Part model, mm, in its own coordinate system. Face numbers are marked on the shaded views. Coordinates: 2 decimals unless noted, no trailing zeros. Order: outer loops, then holes, each group sorted by start corner. A loop starts at its lowest first (then second) coordinate and runs counter-clockwise, first axis right, second up.
1) Cut at D-D (x = 49). List the corners of the cut face in (y, z), and give its area (3 significant figures).
2) Pin check, flat tips, straight feed: pin 1 Ø1.3 at (x, y) = (71, 0) entering from +Z; pin 2 Ø8 at (y, z) = (-3, 16) entering from +X; pin 3 Ø9 at (x, z) = (10, 11) entering from -Y; pin 4 Ø2.5 at (x, z) = (53, 11) entering from -Y. Stop position of each tip, or through.
3) Cut at C-C (z = 11). Give the number of separate pieces and of enclosed holes in the cut face, and give its area (3 significant figures).
4) Wall check: L1, parallel to X at y = -13.5, z = 11; L2, parallel to Z at x = 62, y = 0; L3, parallel to X at y = -11, z = 12. Give the ranges that are in metal, low to high.
5) Cut at B-B (y = 22). List the corners of the cut face in (x, z).
6) Cut at A-A (x = 86). List the corners of the cut face in (y, z).
7) Mould opens along Z. For the marked faces 1, 2 and 3 say: +Z half, -Z half, draft (parallel to the pull), parting line (faces both ways), or undercut.
```python
from build123d import *

# Parameters (mm, degrees)
BOSS_EXTRUDE1_DEPTH     = 90
SKETCH2_R               = 7.6
SKETCH2_R_2             = 5.5
CUT_EXTRUDE1_DEPTH      = 90
SKETCH3_R               = 4.1
CUT_EXTRUDE2_DEPTH      = 90
SKETCH10_W              = 1
SKETCH10_H              = 31.35052841
CUT_EXTRUDE_THIN1_DEPTH = 70
SKETCH11_R              = 11.5
CUT_EXTRUDE6_DEPTH      = 7
SKETCH12_R              = 1.95
CUT_EXTRUDE7_DEPTH      = 15
BOSS_EXTRUDE2_START     = -3
SKETCH16_R              = 4.1
BOSS_EXTRUDE2_DEPTH     = 3
FILLET1_R               = 2
SKETCH17_R              = 2.5
CUT_EXTRUDE8_DEPTH      = 30
SKETCH18_W              = 5
SKETCH18_H              = 7.5
CUT_EXTRUDE9_DEPTH      = 44
BOSS_EXTRUDE3_START     = 3
SKETCH19_R              = 3.5
SKETCH19_R_2            = 2.5
BOSS_EXTRUDE3_DEPTH     = 3
CHAMFER1_SIZE           = 3


with BuildPart() as part:
    # Sketch1 → Boss-Extrude1 (new body)
    with BuildSketch(Plane(origin=(0, 0, 0), x_dir=(0, 0, -1), z_dir=(1, 0, 0))):
        with BuildLine():
            Line((-20, -30), (20, -30))
            ThreePointArc((20, -30), (23.535533906, -28.535533906), (25, -25))
            Line((25, -25), (25, 25))
            ThreePointArc((25, 25), (23.535533906, 28.535533906), (20, 30))
            Line((20, 30), (-20, 30))
            ThreePointArc((-20, 30), (-23.535533906, 28.535533906), (-25, 25))
            Line((-25, 25), (-25, -25))
            ThreePointArc((-25, -25), (-23.535533906, -28.535533906), (-20, -30))
        make_face()
    extrude(amount=BOSS_EXTRUDE1_DEPTH)

    # Sketch2 → Cut-Extrude1 (cut)
    with BuildSketch(Plane(origin=(0, 30, 0), x_dir=(1, 0, 0), z_dir=(0, 1, 0))):
        with Locations(Location((10, -11, 0), (0, 0, 270))):
            Circle(SKETCH2_R)
        with Locations(Location((80, -11, 0), (0, 0, 270))):
            Circle(SKETCH2_R)
        with Locations(Location((45, -11, 0), (0, 0, 270))):
            Circle(SKETCH2_R_2)
    extrude(amount=-CUT_EXTRUDE1_DEPTH, mode=Mode.SUBTRACT)

    # Sketch3 → Cut-Extrude2 (cut)
    with BuildSketch(Plane.XY.offset(25)):
        with Locations((20, 0)):
            Circle(SKETCH3_R)
        with Locations((70, 0)):
            Circle(SKETCH3_R)
    extrude(amount=-CUT_EXTRUDE2_DEPTH, mode=Mode.SUBTRACT)

    # Sketch10 → Cut-Extrude-Thin1 (cut)
    with BuildSketch(Plane(origin=(0, 30, 0), x_dir=(1, 0, 0), z_dir=(0, 1, 0))):
        with Locations((10, -26.675264205)):
            Rectangle(SKETCH10_W, SKETCH10_H)
        with Locations((80, -26.675264205)):
            Rectangle(SKETCH10_W, SKETCH10_H)
    extrude(amount=-CUT_EXTRUDE_THIN1_DEPTH, mode=Mode.SUBTRACT)

    # Sketch11 → Cut-Extrude6 (cut)
    with BuildSketch(Plane(origin=(0, -30, 0), x_dir=(-1, 0, 0), z_dir=(0, -1, 0))):
        with Locations(Location((-45, -11, 0), (0, 0, 90))):
            Circle(SKETCH11_R)
    extrude(amount=-CUT_EXTRUDE6_DEPTH, mode=Mode.SUBTRACT)

    # Sketch12 → Cut-Extrude7 (cut)
    with BuildSketch(Plane(origin=(0, -23, 0), x_dir=(-1, 0, 0), z_dir=(0, -1, 0))):
        with Locations(Location((-45, -19, 0), (0, 0, 90))):
            Circle(SKETCH12_R)
        with Locations(Location((-53, -11, 0), (0, 0, 90))):
            Circle(SKETCH12_R)
        with Locations(Location((-45, -3, 0), (0, 0, 90))):
            Circle(SKETCH12_R)
        with Locations(Location((-37, -11, 0), (0, 0, 90))):
            Circle(SKETCH12_R)
    extrude(amount=-CUT_EXTRUDE7_DEPTH, mode=Mode.SUBTRACT)

    # Sketch16 → Boss-Extrude2 (add)
    with BuildSketch(Plane(origin=(0, 0, -25), x_dir=(-1, 0, 0), z_dir=(0, 0, -1)).offset(BOSS_EXTRUDE2_START)):
        with Locations(Location((-70, 0, 0), (0, 0, 180))):
            Circle(SKETCH16_R)
        with Locations(Location((-20, 0, 0), (0, 0, 180))):
            Circle(SKETCH16_R)
    extrude(amount=BOSS_EXTRUDE2_DEPTH)

    # Fillet1
    fillet1_edges = [part.edges().sort_by_distance(p)[0] for p in [
        (65.9, 0, -22),
        (15.9, 0, -22),
    ]]
    fillet(fillet1_edges, radius=FILLET1_R)

    # Sketch17 → Cut-Extrude8 (cut)
    with BuildSketch(Plane(origin=(90, 0, 0), x_dir=(0, 0, -1), z_dir=(1, 0, 0))):
        Circle(SKETCH17_R)
    extrude(amount=-CUT_EXTRUDE8_DEPTH, mode=Mode.SUBTRACT)

    # Sketch18 → Cut-Extrude9 (cut)
    with BuildSketch(Plane(origin=(0, 30, 0), x_dir=(1, 0, 0), z_dir=(0, 1, 0))):
        with Locations((58.5, 0)):
            Rectangle(SKETCH18_W, SKETCH18_H)
    extrude(amount=-CUT_EXTRUDE9_DEPTH, mode=Mode.SUBTRACT)

    # Sketch19 → Boss-Extrude3 (add)
    with BuildSketch(Plane(origin=(90, 0, 0), x_dir=(0, 0, -1), z_dir=(1, 0, 0)).offset(BOSS_EXTRUDE3_START)):
        with Locations(Location((0, 0, 0), (0, 0, 180))):
            Circle(SKETCH19_R)
        Circle(SKETCH19_R_2, mode=Mode.SUBTRACT)
    extrude(amount=-BOSS_EXTRUDE3_DEPTH)

    # Chamfer1
    chamfer1_edges = [part.edges().sort_by_distance(p)[0] for p in [
        (90, 0, -3.5),
    ]]
    chamfer(chamfer1_edges, length=CHAMFER1_SIZE - 0.0001)  # a hair under: the kernel refuses the full size


solid = part.part
```
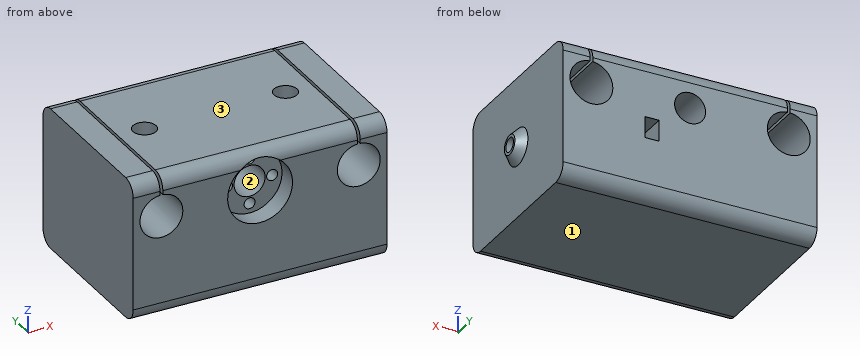
Geometry check:
1. outline: (-30, -20) arc R5 ccw to (-25, -25) - (25, -25) arc R5 ccw to (30, -20) - (30, 7.23) - (-23, 7.23) - (-23, 0.22) - (-30, 0.22) - close; (-29.67, 21.78) - (-23, 21.78) - (-23, 14.77) - (30, 14.77) - (30, 20) arc R5 ccw to (25, 25) - (-25, 25) arc R5 ccw to start
1. area: 2,430 mm2
2. pin 1: stops at z = -22
2. pin 2: stops at x = 90
2. pin 3: passes through
2. pin 4: stops at y = -8
3. separate pieces: 4
3. enclosed holes: 0
3. area: 2,630 mm2
4. L1: x = 0 to 2.4, 17.6 to 35.05, 38.95 to 39.5, 50.5 to 51.05, 54.95 to 72.4, 87.6 to 90
4. L2: z = -25 to -2.5, 2.5 to 25
4. L3: x = 0 to 2.47, 17.53 to 35.33, 38.67 to 39.59, 50.41 to 51.33, 54.67 to 72.47, 87.53 to 90
5. outline: (0, -25) - (90, -25) - (90, 25) - (80.5, 25) - (80.5, 18.58) arc R7.6 cw (long way) to (79.5, 18.58) - (79.5, 25) - (10.5, 25) - (10.5, 18.58) arc R7.6 cw (long way) to (9.5, 18.58) - (9.5, 25) - (0, 25) - close; hole circle Ø11 at (45, 11); hole (56, -3.75) - (61, -3.75) - (61, 3.75) - (56, 3.75) - close
6. outline: (-30, -20) arc R5 ccw to (-25, -25) - (25, -25) arc R5 ccw to (30, -20) - (30, 6.34) - (-30, 6.34) - close; (-30, 15.66) - (30, 15.66) - (30, 20) arc R5 ccw to (25, 25) - (-25, 25) arc R5 ccw to (-30, 20) - close; hole circle Ø5 at (0, 0)
7. face 1: -Z half
7. face 2: undercut
7. face 3: +Z half
